Read the model definition and answer for the solid it produces. Units are mm, in the model's axes. A direction names the side the tool comes from. Give positions to 0.01 mm unless a question says otherwise; leave off trailing zeros. Loops run counter-clockwise (first coordinate to the right, second up) from the corner with the lowest first, then second, coordinate; pieces in that order, holes last. Notation, with made-up numbers: (60, 85) - (71, 85) arc R33 ccw to (71, 116) - close; hole circle Ø2 at (-22, -11). An arc over 180 degrees is marked (long way). Put each result on its own line as item: value. Start each with the question number.
1. A cutting plane is placed at A-A, the plane y = 11.5. Determine the outline of the cut face in (x, z).
2. For a pull along X with two mould halves and no side action, classify faces 6 (the cylindrical face through (-26.93, 1.34, 0.6)), 7 (the flat face through (23, 17, 25)), 8 (the cylindrical face through (18.07, 16.41, 24.4)) as released by +X, released by -X, zero draft, split by the parting line, or undercut.
3. Given pin 1 Ø6.5 at (x, y) = (21.5, 14) entering from +Z; pin 2 Ø7.5 at (x, z) = (-17.5, 17) entering from -Y, each flat-ended and moving along its own axis, determine where each tip first touches the part or whether it passes through.
4. For faces 1 (the cylindrical face through (18.1, -7.52, 16.87)), 2 (the flat face through (22.542, -7.255, 17.605)), 3 (the cylindrical face through (22.46, 24.4, 24.43)), 4 (the cylindrical face through (-18.67, 15.57, 17.98)), 5 (the flat face through (-19.3, 20, 18.2)), determine the directions among +Z, -Z, +X, -X, +Y, -Y from which every point of the face is accessible in a straight line to the end or side of a thin tool.
5. Consider L1, parallel to Z at x = -20.5, y = 7; L2, parallel to Z at x = 25.5, y = 16; L3, parallel to X at y = 3, z = 11.5. Determine where each line is inside the solid, lowest interval first. Write a range as from..to.
6. A cutting plane is placed at B-B, the plane x = 1. Determine the outline of the cut face in (y, z), plus the area to 3 significant figures.
7. A cutting plane is placed at D-D, the plane y = 21. Determine the outline of the cut face in (x, z).
8. A cutting plane is placed at C-C, the plane z = 20.5. Count the separate pieces of the cut face and the enclosed holes in it, plus the area to 3 significant figures.
```python
from build123d import *

# Parameters (mm, degrees)
F0_W     = 55
F0_H     = 50
F1_DEPTH = 10
F5_DEPTH = 10
F6_DEPTH = 10
F7_DEPTH = 10
F8_R     = 2


with BuildPart() as f1:
    # F0 (on Top) → F1 (new body)
    with BuildSketch(Plane.XY):
        Rectangle(F0_W, F0_H)
    extrude(amount=F1_DEPTH)

    # F4 (on face) → F5 (join)
    with BuildSketch(Plane.YZ.offset(27.5)):
        Polygon((-25, 10), (25, 10), (25, 25), (10, 25), align=None)
    extrude(amount=-F5_DEPTH)

    # F3 (on face) → F6 (join)
    with BuildSketch(Plane(origin=(0, 25, 0), x_dir=(-1, 0, 0), z_dir=(0, 1, 0))):
        Polygon((7.5, 10), (27.5, 10), (7.5, 30), align=None)
    extrude(amount=-F6_DEPTH)

    # F2 (on face) → F7 (join)
    with BuildSketch(Plane.XZ.offset(25)):
        Polygon((-27.5, 25), (-27.5, 10), (-2.5, 10), align=None)
    extrude(amount=-F7_DEPTH)

    # F8
    f8_edges = [f1.edges().sort_by_distance(p)[0] for p in [
        (17.5, 25, 17.5),
        (17.5, 17.5, 25),
        (22.5, 25, 25),
        (27.5, 25, 12.5),
        (27.5, 17.5, 25),
        (17.5, -7.5, 17.5),
        (27.5, -7.5, 17.5),
        (-17.5, 25, 20),
        (-17.5, 15, 20),
        (-7.5, 20, 30),
        (-7.5, 25, 20),
        (5, 25, 10),
        (-7.5, 15, 20),
        (-27.5, 0, 0),
        (-27.5, -15, 17.5),
        (-15, -15, 17.5),
        (-27.5, -20, 25),
        (-27.5, -25, 12.5),
        (-15, -25, 17.5),
        (0, -25, 0),
        (27.5, -25, 5),
        (27.5, 0, 0),
        (0, 25, 0),
    ]]
    fillet(f8_edges, radius=F8_R)


solid = f1.part
```
Return value:
1. outline: (-27.5, 2) arc R2 ccw to (-25.5, 0) - (25.5, 0) arc R2 ccw to (27.5, 2) - (27.5, 23) arc R2 ccw to (25.5, 25) - (19.5, 25) arc R2 ccw to (17.5, 23) - (17.5, 10) - (-27.5, 10) - close
2. face 6: released by -X
2. face 7: zero draft
2. face 8: undercut
3. pin 1: stops at z = 25
3. pin 2: stops at y = -25
4. face 1: +Z, -Y
4. face 2: +Z, +X, -Y
4. face 3: +Z, +X, +Y
4. face 4: +Z, -X
4. face 5: +Z, -X, +Y
5. L1: z = 0..10
5. L2: z = 0..25
5. L3: x = 17.5..27.5
6. outline: (-25, 2) arc R2 ccw to (-23, 0) - (23, 0) arc R2 ccw to (25, 2) - (25, 8) arc R2 ccw to (23, 10) - (-25, 10) - close
6. area: 497 mm2
7. outline: (-27.5, 2) arc R2 ccw to (-25.5, 0) - (25.5, 0) arc R2 ccw to (27.5, 2) - (27.5, 23) arc R2 ccw to (25.5, 25) - (19.5, 25) arc R2 ccw to (17.5, 23) - (17.5, 10) - (-7.5, 10) - (-7.5, 25.17) arc R2 ccw to (-10.91, 26.59) - (-27.5, 10) - close
8. separate pieces: 3
8. enclosed holes: 0
8. area: 410 mm2
